Part model, mm, in its own coordinate system. Face numbers are marked on the shaded views. A direction names the side the tool comes from. Round coordinates to 2 decimals unless told otherwise and drop trailing zeros. Loops run counter-clockwise (first coordinate to the right, second up) from the corner with the lowest first, then second, coordinate; pieces in that order, holes last. Notation, with made-up numbers: (27.5, 48.5) - (50.5, 48.5) arc R21 ccw to (50.5, 65.5) - close; hole circle Ø8 at (74, 46). An arc over 180 degrees is marked (long way). Write each question's results on one line, items separated by ' | '. Start each with the question number.
(1) Tool access for the marked faces 5, 6 and 7: list every direction of +Z, -Z, +X, -X, +Y, -Y with a clear straight run to the whole face (end or side of a thin tool).
(2) Flat gauge pins, fed straight in: P1, Ø1, axis at x = -2, y = 2.5, coming from the +Z side; P2, Ø10, axis at y = -3, z = 80, coming from the -X side; P3, Ø3.5, axis at x = -2, z = -23, coming from the -Y side; P4, Ø8, axis at y = -7, z = -29, coming from the +X side. Where does each tip first touch, or does it go through?
(3) Drill centre lines: L1, parallel to X at y = -16, z = -118; L2, parallel to Y at x = -6, z = -76.5; L3, parallel to Z at x = -3, y = -2.5. Where is each one in solid material? Low to high.
(4) Cut at A-A, the plane z = -120. List the corners of the cut face in (x, y).
(5) Cut at B-B, the plane x = 0. Give the number of separate pieces and of enclosed holes in the cut face, then the cut area to 3 significant figures.
(6) Mould opens along Y. For the marked faces 1, 2, 3 and 4 say: released by +Y, released by -Y, zero draft, split by the parting line, or undercut.
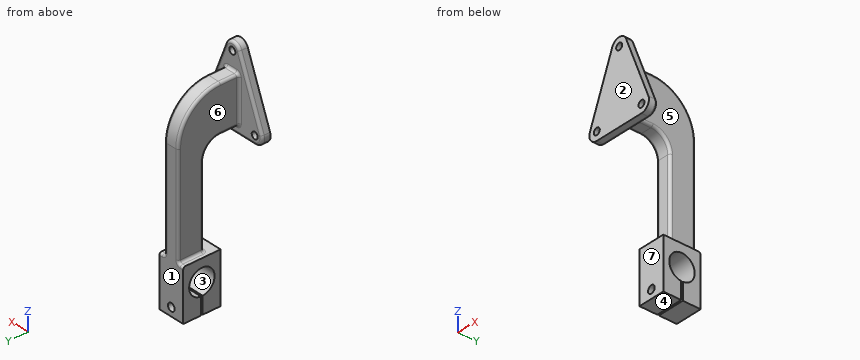
from build123d import *

# Parameters (mm, degrees)
BOSS_EXTRUDE1_DEPTH = 9
SKETCH2_W           = 32
SKETCH2_H           = 44
BOSS_EXTRUDE2_DEPTH = 60
SKETCH3_R           = 15
CUT_EXTRUDE1_DEPTH  = 60
SKETCH4_W           = 34.378885512
SKETCH4_H           = 2
CUT_EXTRUDE2_DEPTH  = 162.300673762
SKETCH5_R           = 4.5
CUT_EXTRUDE3_DEPTH  = 168.593584979
SKETCH6_R           = 4
BOSS_EXTRUDE3_DEPTH = 10
FILLET1_R           = 3


with BuildPart() as part:
    # Sketch1 → Boss-Extrude1 (new, symmetric)
    with BuildSketch(Plane(origin=(0, 0, 0), x_dir=(0, 0, -1), z_dir=(1, 0, 0))):
        with BuildLine():
            Line((90.49122807, -6.438596491), (-4.50877193, -6.438596491))
            ThreePointArc((-4.50877193, -6.438596491), (-18.650907554, -12.296460867), (-24.50877193, -26.438596491))
            Line((-24.50877193, -26.438596491), (-24.50877193, -48.438596491))
            Line((-24.50877193, -48.438596491), (-79.50877193, -48.438596491))
            Line((-79.50877193, -48.438596491), (-79.50877193, -37.438596491))
            Line((-79.50877193, -37.438596491), (-79.50877193, -26.438596491))
            ThreePointArc((-79.50877193, -26.438596491), (-64.864110989, 8.916742568), (-29.50877193, 23.561403509))
            Line((-29.50877193, 23.561403509), (90.49122807, 23.561403509))
            Line((90.49122807, 23.561403509), (90.49122807, -6.438596491))
        make_face()
    extrude(amount=BOSS_EXTRUDE1_DEPTH, both=True)

    # Sketch2 → Boss-Extrude2 (add)
    with BuildSketch(Plane(origin=(0, 0, -90.49122807), x_dir=(-1, 0, 0), z_dir=(0, 0, -1))):
        with Locations((0, 1.561403509)):
            Rectangle(SKETCH2_W, SKETCH2_H)
    extrude(amount=BOSS_EXTRUDE2_DEPTH)

    # Sketch3 → Cut-Extrude1 (cut)
    with BuildSketch(Plane(origin=(16, 0, 0), x_dir=(0, 0, -1), z_dir=(1, 0, 0))):
        with Locations((115.49122807, 1.561403509)):
            Circle(SKETCH3_R)
    extrude(amount=-CUT_EXTRUDE1_DEPTH, mode=Mode.SUBTRACT)

    # Sketch4 → Cut-Extrude2 (cut, through all)
    with BuildSketch(Plane(origin=(16, 0, 0), x_dir=(0, 0, -1), z_dir=(1, 0, 0))):
        with Locations((143.677522108, 1.561403509)):
            Rectangle(SKETCH4_W, SKETCH4_H)
    extrude(amount=-CUT_EXTRUDE2_DEPTH, mode=Mode.SUBTRACT)

    # Sketch5 → Cut-Extrude3 (cut, through all)
    with BuildSketch(Plane(origin=(0, 23.561403509, 0), x_dir=(1, 0, 0), z_dir=(0, 1, 0))):
        with Locations(Location((0, 140.49122807, 0), (0, 0, 270))):
            Circle(SKETCH5_R)
    extrude(amount=-CUT_EXTRUDE3_DEPTH, mode=Mode.SUBTRACT)

    # Sketch6 → Boss-Extrude3 (add)
    with BuildSketch(Plane.XZ.offset(48.438596491)):
        with BuildLine():
            Line((-30, 14.50877193), (30, 14.50877193))
            ThreePointArc((30, 14.50877193), (38.280672305, 18.902483837), (39.284766909, 28.222678693))
            Line((39.284766909, 28.222678693), (9.284766909, 103.222678693))
            ThreePointArc((9.284766909, 103.222678693), (0, 109.50877193), (-9.284766909, 103.222678693))
            Line((-9.284766909, 103.222678693), (-39.284766909, 28.222678693))
            ThreePointArc((-39.284766909, 28.222678693), (-38.280672305, 18.902483837), (-30, 14.50877193))
        make_face()
        with Locations(Location((30, 24.50877193, 0), (0, 0, 270))):
            Circle(SKETCH6_R, mode=Mode.SUBTRACT)
        with Locations(Location((-30, 24.50877193, 0), (0, 0, 270))):
            Circle(SKETCH6_R, mode=Mode.SUBTRACT)
        with Locations(Location((0, 99.50877193, 0), (0, 0, 270))):
            Circle(SKETCH6_R, mode=Mode.SUBTRACT)
    extrude(amount=BOSS_EXTRUDE3_DEPTH)

    # Fillet1
    fillet1_edges = [part.edges().sort_by_distance(p)[0] for p in [
        (9, 8.916742568, 64.864110989),
        (-9, -37.438596491, 79.50877193),
        (-9, 8.916742568, 64.864110989),
        (-9, 23.561403509, -30.49122807),
        (-9, 8.561403509, -90.49122807),
        (-38.280672305, -48.438596491, 18.902483837),
        (0, -48.438596491, 14.50877193),
        (38.280672305, -48.438596491, 18.902483837),
        (24.284766909, -48.438596491, 65.722678693),
        (0, -48.438596491, 109.50877193),
        (-24.284766909, -48.438596491, 65.722678693),
        (9, -37.438596491, 79.50877193),
        (0, -6.438596491, -90.49122807),
        (0, -48.438596491, 24.50877193),
        (0, -48.438596491, 79.50877193),
        (9, -48.438596491, 52.00877193),
        (9, -37.438596491, 24.50877193),
        (9, -12.296460867, 18.650907554),
        (9, -6.438596491, -42.99122807),
        (-12.5, 23.561403509, -90.49122807),
        (12.5, 23.561403509, -90.49122807),
        (9, 8.561403509, -90.49122807),
        (9, 23.561403509, -30.49122807),
        (-9, -6.438596491, -42.99122807),
        (-9, -12.296460867, 18.650907554),
        (-9, -37.438596491, 24.50877193),
        (-9, -48.438596491, 52.00877193),
    ]]
    fillet(fillet1_edges, radius=FILLET1_R)


solid = part.part
A:
1) face 5: +Z, +X, +Y | face 6: +Z, -X, +Y | face 7: -Z, +X, -X, -Y
2) P1: z = 70.63 | P2: through | P3: y = -6.44 | P4: x = 9
3) L1: -16 to 16 | L2: -6.44 to 23.56 | L3: -150.49 to -143.85, -137.14 to -129.93, -101.05 to 73.41
4) outline: (-16, -20.44) - (16, -20.44) - (16, -12.74) - (-16, -12.74) - close; (-16, 15.87) - (16, 15.87) - (16, 23.56) - (-16, 23.56) - close
5) separate pieces: 4 | enclosed holes: 0 | area: 9,350 mm2
6) face 1: released by +Y | face 2: released by -Y | face 3: undercut | face 4: zero draft
